```python
from build123d import *

# Parameters (mm, degrees)
F0_R     = 1.5
F0_W     = 54.5
F0_H     = 15
F1_DEPTH = 3.5
F2_R     = 3.5


with BuildPart() as f1:
    # F0 (on Top) → F1 (new body)
    with BuildSketch(Plane.XY):
        Polygon((27.25, -7.5), (33, -7.5), (33, 7.5), (-33, 7.5), (-33, -7.5), (-27.25, -7.5), align=None)
        with Locations((-30, -3.5)):
            Circle(F0_R, mode=Mode.SUBTRACT)
        with Locations((30, -3.5)):
            Circle(F0_R, mode=Mode.SUBTRACT)
        with Locations((0, -15)):
            Rectangle(F0_W, F0_H)
        with Locations((-24.25, -9.5)):
            Circle(F0_R, mode=Mode.SUBTRACT)
        with Locations((24.25, -9.5)):
            Circle(F0_R, mode=Mode.SUBTRACT)
    extrude(amount=F1_DEPTH)

    # F2
    f2_edges = [f1.edges().sort_by_distance(p)[0] for p in [
        (-33, 7.5, 1.75),
        (33, 7.5, 1.75),
        (27.25, -22.5, 1.75),
        (-27.25, -22.5, 1.75),
        (33, -7.5, 1.75),
        (-33, -7.5, 1.75),
    ]]
    fillet(f2_edges, radius=F2_R)


solid = f1.part
```
Design review of the part built by this model. Coordinates are the model's own, in mm. A direction names the side the tool comes from. Coordinates: 2 decimals unless noted, no trailing zeros. Order: outer loops, then holes, each group sorted by start corner. A loop starts at its lowest first (then second) coordinate and runs counter-clockwise, first axis right, second up. Notation, with made-up numbers: (-8.75, 77.5) - (-0.75, 77.5) arc R13 ccw to (-0.75, 82.5) - close; hole circle Ø7 at (24, -8.5). An arc over 180 degrees is marked (long way). One line per question, with ' | ' between items.
Q1. Consider section C-C, the plane y = -6. Give the boundary of the cut face in (x, z).
Answer key:
outline: (-32.37, 0) - (32.37, 0) - (32.37, 3.5) - (-32.37, 3.5) - close
Q2. Consider section A-A, the plane y = -9.5. Give the boundary of the cut face in (x, z).
Answer key:
outline: (-27.25, 0) - (-25.75, 0) - (-25.75, 3.5) - (-27.25, 3.5) - close; (-22.75, 0) - (22.75, 0) - (22.75, 3.5) - (-22.75, 3.5) - close; (25.75, 0) - (27.25, 0) - (27.25, 3.5) - (25.75, 3.5) - close
Q3. Consider section B-B, the plane z = 2.5. Give the boundary of the cut face in (x, y).
Answer key:
outline: (-33, -4) arc R3.5 ccw to (-29.5, -7.5) - (-27.25, -7.5) - (-27.25, -19) arc R3.5 ccw to (-23.75, -22.5) - (23.75, -22.5) arc R3.5 ccw to (27.25, -19) - (27.25, -7.5) - (29.5, -7.5) arc R3.5 ccw to (33, -4) - (33, 4) arc R3.5 ccw to (29.5, 7.5) - (-29.5, 7.5) arc R3.5 ccw to (-33, 4) - close; hole circle Ø3 at (-30, -3.5); hole circle Ø3 at (-24.25, -9.5); hole circle Ø3 at (24.25, -9.5); hole circle Ø3 at (30, -3.5)
Q4. The part is to be moulded in two halves that separate along Y. For faces 4 (the flat face through (0, -7, 0)), 5 (the cylindrical face through (28.5, -3.43, 1.73)), 6 (the cylindrical face through (32, -6.45, 1.77)), 7 (the cylindrical face through (-31.5, -3.43, 1.73)), say which applies: +Y half, -Y half, draft (parallel to the pull), parting line (faces both ways), or undercut.
Answer key:
face 4: draft | face 5: undercut | face 6: -Y half | face 7: undercut
Q5. For faces 1 (the cylindrical face through (32, 6.45, 1.77)), 2 (the flat face through (27.25, -13, 2)), 3 (the flat face through (-28, -7.5, 2)), list the 3-axis set-ups (+Z, -Z, +X, -X, +Y, -Y) from which the entire face can be reached by the end or side of a thin tool; tool diameter is ignored.
Answer key:
face 1: +Z, -Z, +X, +Y | face 2: +Z, -Z, +X, -Y | face 3: +Z, -Z, -X, -Y
Q6. To check wall thickness, follow line 1 along X through (y, z) = (-2.25, 1.95); line 2 along X through (y, z) = (-4, 2.85); line 3 along Y through (x, z) = (27.5, 1.2). State the ranges of each line that lie inside material, in increasing order.
Answer key:
line 1: x = -33 to -30.83, -29.17 to 29.17, 30.83 to 33 | line 2: x = -33 to -31.41, -28.59 to 28.59, 31.41 to 33 | line 3: y = -7.5 to 7.5
Q7. Clearance check with flat-ended pins moving along their axes: pin 1 Ø1 at (y, z) = (-11.5, 2.5) entering from -X; pin 2 Ø2.5 at (x, y) = (-30, -3.5) entering from +Z; pin 3 Ø1.8 at (x, z) = (28.5, 2) entering from -Y. State where each tip first meets the part, or that it passes through.
Answer key:
pin 1: stops at x = -27.25 | pin 2: passes through | pin 3: stops at y = -7.5
